Geometry: final body of the model. Coordinates: model frame, mm. Give positions to 0.01 mm unless a question says otherwise; leave off trailing zeros. Write each loop counter-clockwise with the first axis right and the second up, starting at its lowest first coordinate (ties: lowest second). Pieces come first, ordered by that corner, then holes.
Q1. Section B-B (z = 20.8). Return the cut outline in (x, y).
Q2. Section D-D (x = -3). Return the cut outline in (y, z).
Q3. Section C-C (y = 2.5). Return the cut outline in (x, z).
Q4. Line query: line 1 (Y direction, x = 2.5, z = 20.9); line 2 (X direction, y = 4.25, z = 20.45); line 3 (X direction, y = 2.25, z = 21.2). Output: solid intervals per line, ascending.
Q5. Pin query (flat end, axial travel): pin 1 Ø2.5 at (x, y) = (2.5, 3) entering from -Z. Return the tip coordinate at first contact, or that it passes through.
Q6. Section A-A (y = -3). Return the cut outline in (x, z), plus the area to 3 significant figures.
Q7. Mould query, pull axis X, two halves, no side actions, for faces 1 (the cylindrical face through (-5, 0, 21)), 2 (the flat face through (15, -7.5, 21)), 3 (the cylindrical face through (2.305, 1.513, 20.986)). Classes: +X half, -X half, draft (parallel to the pull), parting line (faces both ways), or undercut.
Autodesk Inventor part; units mm, degrees
ref_plane "Work Plane1" through (0, 0, 20) normal (0, 0, 1) x (1, 0, 0)
ref_plane "YZ Plane" through (0, 0, 0) normal (1, 0, 0) x (0, 1, 0)
ref_plane "XZ Plane" through (0, 0, 0) normal (0, 1, 0) x (-1, 0, 0)
sketch "Sketch1" plane through (0, 0, 0) normal (0, 0, 1) x (1, 0, 0)
  circle A0 centre (0, 0) radius 11.25
  line L0 (0, 0) -> (2.5, 0)
  circle A1 centre (2.5, 0) radius 7.5
  line L1 (8, 6.7455) -> (8, -7.7933)
  point P0 (10, 0)
  point P1 (10, 0)
  point P2 (8, -5.099)
  point P3 (8, 5.099)
  dimension "d2" = 15
  dimension "d0" = 22.5
  dimension "d1" = 2.5
  dimension "d3" = 2
extrude "Extrusion1" [suppressed]
extrude "Extrusion2" [suppressed]
sketch "Sketch2" plane through (2.5, 0, 13.5) normal (0, 0, 1) x (1, 0, 0)
  line L0 (0, 0) -> (0, 3)
  circle A0 centre (0, 3) radius 2.75
  line L1 (-18.25, 0) -> (13.25, 0) construction
  circle A1 centre (0, -3) radius 2.75
  point P0 (-2.5, 0)
  dimension "d8" = 3
  dimension "d23" = 5.5
hole "Hole1" [suppressed]
feature "FaceDraft1" [suppressed]
ref_plane "Work Plane1" through (0, 0, 20) normal (0, 0, 1) x (1, 0, 0)
sketch "Sketch3" plane through (0, 0, 20) normal (0, 0, 1) x (1, 0, 0)
  arc A0 (8, 5.099) -> (8, -5.099) centre (2.5, 0) ccw
  circle A1 centre (2.5, 3) radius 1.5
  line L0 (2.5, 7.5) -> (27.5, 7.5)
  line L1 (2.5, -7.5) -> (27.5, -7.5)
  line L2 (27.5, -7.5) -> (27.5, 7.5)
  circle A2 centre (2.5, -3) radius 1.5
  point P0 (0, 0)
  dimension "d18" = 25
  dimension "d19" = 25
extrude "Extrusion3" add sketch "Sketch3" along normal blind 2
properties part number "Leaver"
Computed:
1. outline: (2.5, -7.5) - (27.5, -7.5) - (27.5, 7.5) - (2.5, 7.5) arc R7.5 ccw to start; hole circle Ø3 at (2.5, -3); hole circle Ø3 at (2.5, 3)
2. outline: (-5.1, 20) - (5.1, 20) - (5.1, 22) - (-5.1, 22) - close
3. outline: (-4.57, 20) - (1.09, 20) - (1.09, 22) - (-4.57, 22) - close; (3.91, 20) - (27.5, 20) - (27.5, 22) - (3.91, 22) - close
4. line 1: y = -7.5 to -4.5, -1.5 to 1.5, 4.5 to 7.5
4. line 2: x = -3.68 to 1.67, 3.33 to 27.5
4. line 3: x = -4.65 to 1.2, 3.8 to 27.5
5. pin 1: passes through
6. outline: (-4.37, 20) - (1, 20) - (1, 22) - (-4.37, 22) - close; (4, 20) - (27.5, 20) - (27.5, 22) - (4, 22) - close
6. area: 57.7 mm2
7. face 1: -X half
7. face 2: draft
7. face 3: undercut
